Check sheet for the modelled part. Datum: model origin and axes. Units: mm. A direction names the side the tool comes from. Give positions to 0.01 mm unless a question says otherwise; leave off trailing zeros. Answer in a Markdown table with one row per item.
from build123d import *

# Parameters (mm, degrees)
F2_DEPTH = 2.5
F1_R     = 2.5
F3_DEPTH = 2.5
F5_DEPTH = 2.5
F4_W     = 30
F4_H     = 2
F6_DEPTH = 2.5
F7_DEPTH = 2.5


with BuildPart() as f2:
    # F0 (on Front) → F2 (new body)
    with BuildSketch(Plane.XZ):
        with BuildLine():
            add(Edge.make_bspline(
                [(-96.9805282175, -0.8100506688), (-84.7869920978, 5.1468541776), (-38.6381415733, 10.9636146396), (42.6881882799, 2.4723259958), (100, -4.047003109)],
                knots=[0, 0, 0, 0, 0.374886421, 1, 1, 1, 1], degree=3))
            add(Edge.make_bspline(
                [(-97.5447368223, -7.1186651935), (-99.939251346, -6.5508492693), (-102.885147974, -5.168950634), (-100.0067471137, -2.3789404522), (-96.9805282175, -0.8100506688)],
                knots=[0.0564585679, 0.0564585679, 0.0564585679, 0.0564585679, 0.4847104148, 1, 1, 1, 1], degree=3))
            add(Edge.make_bspline(
                [(-96.5428845142, -7.3406707446), (-96.8949965543, -7.2673488468), (-97.22905608, -7.1935231869), (-97.5447368223, -7.1186651935)],
                knots=[0, 0, 0, 0, 0.0564585679, 0.0564585679, 0.0564585679, 0.0564585679], degree=3))
            add(Edge.make_bspline(
                [(-96.5428845142, -7.3406707446), (-80.7020161693, -9.4302402111), (-44.2471235075, -11.1181020976), (41.8622965332, -3.5518856086), (82.0915186506, -4.6802794425), (100, -4.047003109)],
                knots=[0, 0, 0, 0, 0.2987594418, 0.6837410955, 1, 1, 1, 1], degree=3))
        make_face()
        with BuildLine():
            add(Edge.make_bspline(
                [(-99.8196757147, -4.047003109), (-99.3821638101, -3.2227137691), (-97.9006497107, -2.3042858417), (-96.3385477662, -1.6362179573)],
                knots=[0.5425000514, 0.5425000514, 0.5425000514, 0.5425000514, 1, 1, 1, 1], degree=3))
            add(Edge.make_bspline(
                [(-96.3385477662, -1.6362179573), (-85.7442874691, 3.2900694446), (-38.7960585931, 10.0747672146), (36.943279708, 1.696590452), (86.094097513, -3.3751911245)],
                knots=[0, 0, 0, 0, 0.384923117, 1, 1, 1, 1], degree=3))
            add(Edge.make_bspline(
                [(-97.3825784566, -6.0471531808), (-82.3468325761, -8.841713568), (-44.2551066449, -8.6286827794), (40.9195716837, -3.3120714751), (72.7341022162, -3.1550192186), (86.094097513, -3.3751911245)],
                knots=[0, 0, 0, 0, 0.3131273629, 0.7122131732, 1, 1, 1, 1], degree=3))
            add(Edge.make_bspline(
                [(-97.3825784566, -6.0471531808), (-98.6588937786, -5.8946130057), (-100.1661659123, -5.1778479876), (-99.9138553768, -4.2244412327), (-99.8196757147, -4.047003109)],
                knots=[0, 0, 0, 0, 0.4440177242, 0.5425000514, 0.5425000514, 0.5425000514, 0.5425000514], degree=3))
        make_face(mode=Mode.SUBTRACT)
        with BuildLine():
            add(Edge.make_bspline(
                [(-96.3385477662, -1.6362179573), (-85.7442874691, 3.2900694446), (-38.7960585931, 10.0747672146), (36.943279708, 1.696590452), (86.094097513, -3.3751911245)],
                knots=[0, 0, 0, 0, 0.384923117, 1, 1, 1, 1], degree=3))
            add(Edge.make_bspline(
                [(-99.8196757147, -4.047003109), (-99.3821638101, -3.2227137691), (-97.9006497107, -2.3042858417), (-96.3385477662, -1.6362179573)],
                knots=[0.5425000514, 0.5425000514, 0.5425000514, 0.5425000514, 1, 1, 1, 1], degree=3))
            add(Edge.make_bspline(
                [(-97.3825784566, -6.0471531808), (-98.6588937786, -5.8946130057), (-100.1661659123, -5.1778479876), (-99.9138553768, -4.2244412327), (-99.8196757147, -4.047003109)],
                knots=[0, 0, 0, 0, 0.4440177242, 0.5425000514, 0.5425000514, 0.5425000514, 0.5425000514], degree=3))
            add(Edge.make_bspline(
                [(-97.3825784566, -6.0471531808), (-82.3468325761, -8.841713568), (-44.2551066449, -8.6286827794), (40.9195716837, -3.3120714751), (72.7341022162, -3.1550192186), (86.094097513, -3.3751911245)],
                knots=[0, 0, 0, 0, 0.3131273629, 0.7122131732, 1, 1, 1, 1], degree=3))
        make_face()
        with BuildLine():
            add(Edge.make_bspline(
                [(-96.5428845142, -7.3406707446), (-96.8949965543, -7.2673488468), (-97.22905608, -7.1935231869), (-97.5447368223, -7.1186651935)],
                knots=[0, 0, 0, 0, 0.0564585679, 0.0564585679, 0.0564585679, 0.0564585679], degree=3))
            ThreePointArc((-97.5447368223, -7.1186651935), (-97.052492706, -7.2688477084), (-96.5428845142, -7.3406707446))
        make_face()
    extrude(amount=F2_DEPTH)


with BuildPart() as f2b:
    # F1 (on Front) → F2, piece 2 (new body)
    with BuildSketch(Plane.XZ):
        with Locations((33.7789729238, -1.0305350879)):
            Circle(F1_R)
    extrude(amount=F2_DEPTH)


with BuildPart() as f2c:
    # F1 (on Front) → F2, piece 3 (new body)
    with BuildSketch(Plane.XZ):
        with BuildLine():
            ThreePointArc((-45.542362095, -1.3708024857), (-51.4789804014, 2.1291274472), (-51.6671168627, -4.7598166753))
            Line((-51.6671168627, -4.7598166753), (-47.385046135, -4.7391830831))
            ThreePointArc((-47.385046135, -4.7391830831), (-46.0331411102, -3.2905337378), (-45.542362095, -1.3708024857))
        make_face()
        with BuildLine():
            Line((-47.385046135, -4.7391830831), (-51.6671168627, -4.7598166753))
            ThreePointArc((-51.6671168627, -4.7598166753), (-49.523087913, -5.3707560487), (-47.385046135, -4.7391830831))
        make_face()
    extrude(amount=F2_DEPTH)


with BuildPart() as f3_tool:
    # F1 (on Front) → F3 (new body)
    with BuildSketch(Plane.XZ):
        with BuildLine():
            ThreePointArc((-45.542362095, -1.3708024857), (-51.4789804014, 2.1291274472), (-51.6671168627, -4.7598166753))
            Line((-51.6671168627, -4.7598166753), (-47.385046135, -4.7391830831))
            ThreePointArc((-47.385046135, -4.7391830831), (-46.0331411102, -3.2905337378), (-45.542362095, -1.3708024857))
        make_face()
        with BuildLine():
            Line((-47.385046135, -4.7391830831), (-51.6671168627, -4.7598166753))
            ThreePointArc((-51.6671168627, -4.7598166753), (-49.523087913, -5.3707560487), (-47.385046135, -4.7391830831))
        make_face()
        with Locations((33.7789729238, -1.0305350879)):
            Circle(F1_R)
    extrude(amount=F3_DEPTH)


with BuildPart() as f2_1:
    add(f2.part)

    # F3: cut by f3_tool
    add(f3_tool.part, mode=Mode.SUBTRACT)

    # F4 (on face) → F5 (cut)
    with BuildSketch(Plane.XZ.offset(2.5)):
        with BuildLine():
            Line((-96.5428845142, -7.3406707446), (-96.5428845142, -0.5989118026))
            add(Edge.make_bspline(
                [(-96.9805282175, -0.8100506688), (-96.8353706427, -0.7391368787), (-96.6894893165, -0.6687582494), (-96.5428845142, -0.5989118026)],
                knots=[0, 0, 0, 0, 0.0044628238, 0.0044628238, 0.0044628238, 0.0044628238], degree=3))
            add(Edge.make_bspline(
                [(-96.9805282175, -0.8100506688), (-100.0067471137, -2.3789404522), (-102.885147974, -5.168950634), (-99.939251346, -6.5508492693), (-97.5447368223, -7.1186651935)],
                knots=[0.0564585679, 0.0564585679, 0.0564585679, 0.0564585679, 0.5717481532, 1, 1, 1, 1], degree=3))
            ThreePointArc((-97.5447368223, -7.1186651935), (-97.052492706, -7.2688477084), (-96.5428845142, -7.3406707446))
        make_face()
    extrude(amount=-F5_DEPTH, mode=Mode.SUBTRACT)

    # F4 (on face) → F6 (cut)
    with BuildSketch(Plane.XZ.offset(2.5)):
        with BuildLine():
            Line((-78.6215588156, -7.3670944992), (-78.6215588156, 3.2958948603))
            add(Edge.make_bspline(
                [(-78.6215588156, 3.2958948603), (-83.9345486349, 2.2532028855), (-88.8194569144, 0.5548157735), (-93.7043651938, -1.1435713386)],
                knots=[0.554896308, 0.554896308, 0.554896308, 0.554896308, 1, 1, 1, 1], degree=3))
            Line((-93.7043651938, -1.1435713386), (-93.7043651938, -6.1954581179))
            add(Edge.make_bspline(
                [(-78.6215588156, -7.3670944992), (-83.7013643272, -7.1077100258), (-88.7028647605, -6.6515840718), (-93.7043651938, -6.1954581179)],
                knots=[0.5793594661, 0.5793594661, 0.5793594661, 0.5793594661, 1, 1, 1, 1], degree=3))
        make_face()
        with BuildLine():
            Line((-57.251535356, -7.4831936508), (-57.251535356, 4.8988820054))
            add(Edge.make_bspline(
                [(-57.251535356, 4.8988820054), (-63.1249518816, 4.7812850577), (-68.9983684072, 4.66368811), (-74.4892291338, 3.9601280834)],
                knots=[0, 0, 0, 0, 0.4418705618, 0.4418705618, 0.4418705618, 0.4418705618], degree=3))
            Line((-74.4892291338, 3.9601280834), (-74.4892291338, -7.5306241193))
            add(Edge.make_bspline(
                [(-57.251535356, -7.4831936508), (-63.0319736557, -7.5857864832), (-68.8124119553, -7.6883793156), (-74.4892291338, -7.5306241193)],
                knots=[0, 0, 0, 0, 0.4658094847, 0.4658094847, 0.4658094847, 0.4658094847], degree=3))
        make_face()
        with Locations((-27.6331795752, 3.8601249214)):
            Rectangle(F4_W, F4_H)
        Polygon((27.7735989974, 1.9125135442), (2.0833725575, 3.8092588075), (2.0833725575, -4.047003109), (27.937149629, -3.2237600535), align=None)
    extrude(amount=-F6_DEPTH, mode=Mode.SUBTRACT)

    # F4 (on face) → F7 (cut)
    with BuildSketch(Plane.XZ.offset(2.5)):
        with BuildLine():
            add(Edge.make_bspline(
                [(62.5460875734, 0.1020588345), (74.6514883615, -1.1873862537), (87.1633646635, -2.586811085), (100, -4.047003109)],
                knots=[0.8599877614, 0.8599877614, 0.8599877614, 0.8599877614, 1, 1, 1, 1], degree=3))
            Line((62.5460875734, 0.1020588345), (62.5460875734, -4.518638291))
            add(Edge.make_bspline(
                [(62.5460875734, -4.518638291), (75.9097127299, -4.3829595873), (88.0075171585, -4.4710790211), (100, -4.047003109)],
                knots=[0.7882160183, 0.7882160183, 0.7882160183, 0.7882160183, 1, 1, 1, 1], degree=3))
        make_face()
    extrude(amount=-F7_DEPTH, mode=Mode.SUBTRACT)


with BuildPart() as f2b_1:
    add(f2b.part)

    # F3: cut by f3_tool
    add(f3_tool.part, mode=Mode.SUBTRACT)


with BuildPart() as f2c_1:
    add(f2c.part)

    # F3: cut by f3_tool
    add(f3_tool.part, mode=Mode.SUBTRACT)


solid = f2_1.part
(1) Thickness scan on L1, parallel to X at y = -1.2, z = -2; L2, parallel to X at y = -0.2, z = -1.75; L3, parallel to Z at x = -50, y = -2.25. Record the ranges inside material, lowest first.
Geometry says:
| item | result |
|---|---|
| L1 | -96.54 to -93.7, -78.62 to -74.49, -57.25 to -53.49, -45.59 to 2.08, 27.9 to 31.47, 36.08 to 62.55 |
| L2 | -96.54 to -93.7, -78.62 to -74.49, -57.25 to -53.52, -45.56 to 2.08, 27.89 to 31.38, 36.17 to 62.55 |
| L3 | -9.72 to -5.34, 2.6 to 7.43 |
(2) Access from +Z, -Z, +X, -X, +Y, -Y to the whole of each face (thin tool, end or side, straight path). Record for faces 4 (the flat face through (-28, -1, 4.86)), 5 (the flat face through (-96.543, -1, -4)).
Geometry says:
| item | result |
|---|---|
| face 4 | +Y, -Y |
| face 5 | +Z, -Z, -X, +Y, -Y |
(3) Mould release check, pull along X, two halves, no side actions. Record for faces 1 (the flat face through (-16, -2.5, 0)), 2 (the flat face through (62.546, -1, -2)), 3 (the cylindrical face through (36.088, -1.232, -1.988)): pulls with the +X half, pulls with the -X half, needs draft (parallel to the pull), parting line crosses it, or undercut.
Geometry says:
| item | result |
|---|---|
| face 1 | needs draft |
| face 2 | pulls with the +X half |
| face 3 | undercut |
(4) Gauge pin test, flat end, axial feed: P1, Ø1.5, axis at x = 17.5, y = -1, coming from the +Z side. Record the tip position at first contact, or that the pin passes through.
Geometry says:
| item | result |
|---|---|
| P1 | z = 4.53 |
(5) Cross-section at A-A, the plane y = -1.45. Give the number of separate pieces and of enclosed holes in the cut face, then the cut area to 3 significant figures.
Geometry says:
| item | result |
|---|---|
| separate pieces | 1 |
| enclosed holes | 6 |
| area | 1,360 mm² |
